Source: CAD feature listing. Evaluate the final solid. Frame: model axes, mm. Give positions to 0.01 mm unless a question says otherwise; leave off trailing zeros. Loops run counter-clockwise (first coordinate to the right, second up) from the corner with the lowest first, then second, coordinate; pieces in that order, holes last.
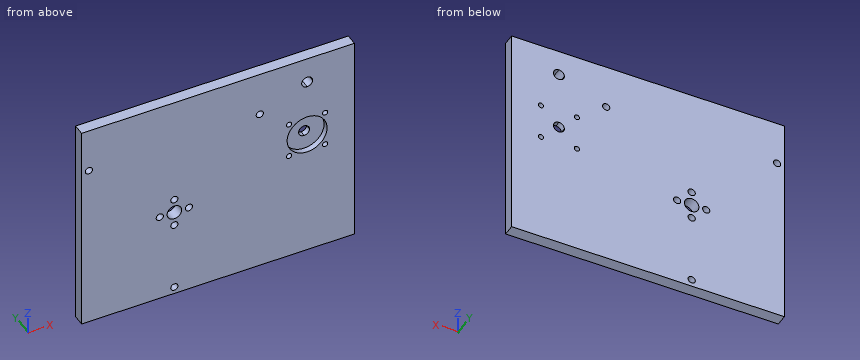
```python
from build123d import *

# Parameters (mm, degrees)
SKETCH1_W           = 150
SKETCH1_H           = 120
BOSS_EXTRUDE1_DEPTH = 6.35
SKETCH2_R           = 2
SKETCH2_R_2         = 4
CUT_EXTRUDE1_DEPTH  = 10
SKETCH3_R           = 11
CUT_EXTRUDE2_DEPTH  = 3.21
SKETCH4_R           = 1.45
CUT_EXTRUDE3_DEPTH  = 6.35


with BuildPart() as part:
    # Sketch1 → Boss-Extrude1 (new body)
    with BuildSketch(Plane(origin=(0, 0, 0), x_dir=(1, 0, 0), z_dir=(0, 1, 0))):
        with Locations((75, 60)):
            Rectangle(SKETCH1_W, SKETCH1_H)
    extrude(amount=BOSS_EXTRUDE1_DEPTH)

    # Sketch2 → Cut-Extrude1 (cut)
    with BuildSketch(Plane(origin=(0, 6.35, 0), x_dir=(1, 0, 0), z_dir=(0, 1, 0))):
        with Locations(Location((51, 116, 0), (0, 0, 270))):
            Circle(SKETCH2_R)
        with Locations(Location((4, 25, 0), (0, 0, 270))):
            Circle(SKETCH2_R)
        with Locations(Location((98, 25, 0), (0, 0, 270))):
            Circle(SKETCH2_R)
        with BuildLine():
            ThreePointArc((127, 14.5), (126.121320344, 16.621320344), (124, 17.5))
            Line((124, 17.5), (124, 14.5))
            Line((124, 14.5), (124, 11.5))
            ThreePointArc((124, 11.5), (126.121320344, 12.378679656), (127, 14.5))
        make_face()
        with BuildLine():
            Line((124, 14.5), (124, 17.5))
            ThreePointArc((124, 17.5), (121.878679656, 16.621320344), (121, 14.5))
            Line((121, 14.5), (124, 14.5))
        make_face()
        with BuildLine():
            Line((124, 14.5), (121, 14.5))
            ThreePointArc((121, 14.5), (121.878679656, 12.378679656), (124, 11.5))
            Line((124, 11.5), (124, 14.5))
        make_face()
        with BuildLine():
            ThreePointArc((121, 47.5), (121.878679656, 45.378679656), (124, 44.5))
            Line((124, 44.5), (124, 47.5))
            Line((124, 47.5), (121, 47.5))
        make_face()
        with BuildLine():
            ThreePointArc((124, 50.5), (121.878679656, 49.621320344), (121, 47.5))
            Line((121, 47.5), (124, 47.5))
            Line((124, 47.5), (124, 50.5))
        make_face()
        with BuildLine():
            Line((124, 47.5), (124, 44.5))
            ThreePointArc((124, 44.5), (126.121320344, 45.378679656), (127, 47.5))
            ThreePointArc((127, 47.5), (126.121320344, 49.621320344), (124, 50.5))
            Line((124, 50.5), (124, 47.5))
        make_face()
        with Locations(Location((51, 77, 0), (0, 0, 270))):
            Circle(SKETCH2_R)
        with Locations(Location((43, 69, 0), (0, 0, 270))):
            Circle(SKETCH2_R)
        with Locations(Location((51, 69, 0), (0, 0, 270))):
            Circle(SKETCH2_R_2)
        with Locations(Location((59, 69, 0), (0, 0, 270))):
            Circle(SKETCH2_R)
        with Locations(Location((51, 61, 0), (0, 0, 270))):
            Circle(SKETCH2_R)
    extrude(amount=-CUT_EXTRUDE1_DEPTH, mode=Mode.SUBTRACT)

    # Sketch3 → Cut-Extrude2 (cut)
    with BuildSketch(Plane.XZ):
        with Locations(Location((124, -47.5, 0), (0, 0, 270))):
            Circle(SKETCH3_R)
    extrude(amount=-CUT_EXTRUDE2_DEPTH, mode=Mode.SUBTRACT)

    # Sketch4 → Cut-Extrude3 (cut)
    with BuildSketch(Plane(origin=(0, 6.35, 0), x_dir=(1, 0, 0), z_dir=(0, 1, 0))):
        with Locations(Location((133.899494937, 57.399494937, 0), (0, 0, 270))):
            Circle(SKETCH4_R)
        with Locations(Location((114.100505063, 37.600505063, 0), (0, 0, 270))):
            Circle(SKETCH4_R)
        with Locations(Location((133.899494937, 37.600505063, 0), (0, 0, 270))):
            Circle(SKETCH4_R)
        with Locations(Location((114.100505063, 57.399494937, 0), (0, 0, 270))):
            Circle(SKETCH4_R)
    extrude(amount=-CUT_EXTRUDE3_DEPTH, mode=Mode.SUBTRACT)


solid = part.part
```
(1) First-contact query: pin 1 (2.5 mm diameter, centred on x = 51, z = -116, fed in from +Y). Flat tip, straight axial feed; report the tip coordinate or a pass-through.
A:
pin 1: passes through
(2) Section A-A, the plane x = 4. Return the cut outline in (y, z), then the cut area to 3 significant figures.
A:
outline: (0, -120) - (6.35, -120) - (6.35, -27) - (0, -27) - close; (0, -23) - (6.35, -23) - (6.35, 0) - (0, 0) - close
area: 737 mm2
(3) Section B-B, the plane z = -61. Return the cut outline in (x, y), then the cut area to 3 significant figures.
A:
outline: (0, 0) - (49, 0) - (49, 6.35) - (0, 6.35) - close; (53, 0) - (150, 0) - (150, 6.35) - (53, 6.35) - close
area: 927 mm2
(4) Ray query, line 1 along X through (y, z) = (2.1, -47.5); line 2 along X through (y, z) = (1.5, -69); line 3 along X through (y, z) = (5.75, -37). Return the intervals inside material, ascending.
A:
line 1: x = 0 to 113, 135 to 150
line 2: x = 0 to 41, 45 to 47, 55 to 57, 61 to 150
line 3: x = 0 to 112.78, 115.42 to 132.58, 135.22 to 150
(5) Section C-C, the plane y = 2. Count the separate pieces of the cut face and the enclosed holes in it, then the cut area to 3 significant figures.
A:
separate pieces: 1
enclosed holes: 14
area: 17,400 mm2
